Check sheet for the modelled part. Datum: model origin and axes. Units: mm. A direction names the side the tool comes from. Coordinates: 2 decimals unless noted, no trailing zeros. Loops run counter-clockwise (first coordinate to the right, second up) from the corner with the lowest first, then second, coordinate; pieces in that order, holes last. Notation, with made-up numbers: (66.25, 60) - (108.25, 60) arc R25 ccw to (108.25, 84) - close; hole circle Ø8 at (34, -0.5). An arc over 180 degrees is marked (long way). Use a Markdown table: item, result. Add a question column.
1) Thickness scan on line 1 (Z direction, x = 26.5, y = -29); line 2 (Y direction, x = 10, z = -35); line 3 (X direction, y = 18.5, z = -11.5). Record the ranges inside material, lowest first.
2) Tool access check on faces 5 (the flat face through (15, 138, -103)), 6 (the flat face through (15, 110, -116)), 7 (the flat face through (2, 51, -8)). Record the directions out of +Z, -Z, +X, -X, +Y, -Y that give a thin tool (end or side, any length) a straight path to the whole face; none if there is none.
3) Sectioned sample at B-B, the plane y = 69. Enter the section's corners in (x, z), then the cut area to 3 significant figures.
4) Sectioned sample at C-C, the plane x = 8. Enter the section's corners in (y, z), then the cut area to 3 significant figures.
5) Sectioned sample at A-A, the plane z = -193. Enter the section's corners in (x, y), then the cut area to 3 significant figures.
6) Draft check along Z on faces 1 (the flat face through (14.82, -122.35, 0.18)), 2 (the flat face through (15, -2, -15)), 3 (the flat face through (15, 3, 13)), 4 (the flat face through (0, 51, -14)). Enter one of: pulls with the +Z half, pulls with the -Z half, needs draft (parallel to the pull), parting line crosses it, or undercut.
7) Go/stop test with flat-tipped pins: P1, Ø9, axis at x = 20, z = -154.5, coming from the -Y side; P2, Ø5, axis at x = 19, y = -57.5, coming from the -Z side. Record where each tip stops, or that it passes through.
from build123d import *

# Parameters (mm, degrees)
F0_W     = 30
F0_H     = 200
F1_DEPTH = 30
F2_T     = -2


with BuildPart() as f1:
    # F0 (on Right) → F1 (new body)
    with BuildSketch(Plane.YZ):
        with Locations((125, -115)):
            Rectangle(F0_W, F0_H)
        Polygon((110, -15), (140, -15), (140, 15), (-140, 15), (-110, -15), align=None)
    extrude(amount=F1_DEPTH)

    # F2
    f2_openings = [f1.faces().sort_by_distance(p)[0] for p in [
        (15, 125, -215),
    ]]
    offset(amount=F2_T, openings=f2_openings, kind=Kind.INTERSECTION)


solid = f1.part
Solved:
| question | item | result |
|---|---|---|
| 1 | line 1 | z = -15 to -13, 13 to 15 |
| 1 | line 2 | y = 110 to 112, 138 to 140 |
| 1 | line 3 | x = 0 to 2, 28 to 30 |
| 2 | face 5 | -Z |
| 2 | face 6 | -Z, +X, -X, -Y |
| 2 | face 7 | none |
| 3 | outline | (0, -15) - (30, -15) - (30, 15) - (0, 15) - close; hole (2, -13) - (28, -13) - (28, 13) - (2, 13) - close |
| 3 | area | 224 mm2 |
| 4 | outline | (-140, 15) - (-110, -15) - (110, -15) - (110, -215) - (112, -215) - (112, -13) - (-109.17, -13) - (-135.17, 13) - (138, 13) - (138, -215) - (140, -215) - (140, 15) - close |
| 4 | area | 1,930 mm2 |
| 5 | outline | (0, 110) - (30, 110) - (30, 140) - (0, 140) - close; hole (2, 112) - (28, 112) - (28, 138) - (2, 138) - close |
| 5 | area | 224 mm2 |
| 6 | face 1 | undercut |
| 6 | face 2 | pulls with the -Z half |
| 6 | face 3 | undercut |
| 6 | face 4 | needs draft |
| 7 | P1 | stops at y = 110 |
| 7 | P2 | stops at z = -15 |
